Autodesk Inventor part; units mm, degrees
ref_plane "YZ Plane" through (0, 0, 0) normal (1, 0, 0) x (0, 1, 0)
ref_plane "XZ Plane" through (0, 0, 0) normal (0, 1, 0) x (-1, 0, 0)
ref_plane "XY Plane" through (0, 0, 0) normal (0, 0, 1) x (1, 0, 0)
sketch "Sketch1" plane through (0, 0, 0) normal (0, 0, 1) x (1, 0, 0)
  point P0 (0, 0)
sketch "0" plane through (0, 0, 0) normal (0, 0, 1) x (1, 0, 0)
  arc A0 (31.9, 54.31) -> (34.9, 51.31) centre (34.9, 54.31) ccw
  line L0 (34.9, 51.31) -> (39.9, 51.31)
  arc A1 (42.9, 48.31) -> (39.9, 51.31) centre (39.9, 48.31) ccw
  line L1 (42.9, 48.31) -> (42.9, 28.56)
  arc A2 (39.9, 25.56) -> (42.9, 28.56) centre (39.9, 28.56) ccw
  line L2 (39.9, 25.56) -> (34.9, 25.56)
  line L3 (15.6769, 19.4231) -> (14.5, 19.4231)
  arc A3 (12.5, 21.4231) -> (14.5, 19.4231) centre (14.5, 21.4231) ccw
  line L4 (12.5, 21.4231) -> (12.5, 22.56)
  arc A4 (12.5, 22.56) -> (9.5, 25.56) centre (9.5, 22.56) ccw
  line L5 (9.5, 51.31) -> (4.5, 51.31)
  arc A5 (4.5, 51.31) -> (1.5, 48.31) centre (4.5, 48.31) ccw
  line L6 (1.5, 48.31) -> (1.5, 28.56)
  arc A6 (1.5, 28.56) -> (4.5, 25.56) centre (4.5, 28.56) ccw
  line L7 (4.5, 25.56) -> (9.5, 25.56)
  arc A7 (31.9, 54.31) -> (28.9, 57.31) centre (28.9, 54.31) ccw
  line L8 (28.9, 57.31) -> (15.5, 57.31)
  arc A8 (15.5, 57.31) -> (12.5, 54.31) centre (15.5, 54.31) ccw
  line L9 (28.7231, 19.4231) -> (29.9, 19.4231)
  arc A9 (29.9, 19.4231) -> (31.9, 21.4231) centre (29.9, 21.4231) ccw
  line L10 (31.9, 21.4231) -> (31.9, 22.56)
  line L11 (12.705, 53.275) -> (12.705, 23.375)
  line L12 (15.805, 56.275) -> (28.595, 56.275)
  line L13 (31.595, 53.275) -> (31.595, 23.375)
  line L14 (30.345, 22.125) -> (14.055, 22.125)
  circle A10 centre (9.5, 54.31) radius 2
  circle A11 centre (9.5, 22.56) radius 2
  circle A12 centre (34.9, 22.56) radius 2
  circle A13 centre (34.9, 54.31) radius 2
  circle A14 centre (9.5, 54.31) radius 3
  circle A15 centre (9.5, 22.56) radius 3
  circle A16 centre (34.9, 22.56) radius 3
  circle A17 centre (34.9, 54.31) radius 3
  circle A18 centre (22.2, 12.9) radius 8.75
  circle A19 centre (22.2, 12.9) radius 9.225
  arc A20 (28.7231, 19.4231) -> (15.6769, 19.4231) centre (22.2, 12.9) ccw
  line L15 (22.2, 12.9) -> (28.7231, 19.4231)
  line L16 (22.2, 12.9) -> (31.425, 12.9)
  line L17 (22.2, 12.9) -> (15.6769, 19.4231)
  arc A21 (9.5, 51.31) -> (12.5, 54.31) centre (9.5, 54.31) ccw
  arc A22 (34.9, 25.56) -> (31.9, 22.56) centre (34.9, 22.56) ccw
  point P0 (31.9, 54.31)
  point P1 (12.5, 54.31)
  point P2 (4.5, 51.31)
  point P3 (1.5, 48.31)
extrude "Extrusion1" add sketch "0" along normal blind 1.5 contours A0 L0 A1 L1 A2 L2 A16 L10 A9 L9 A19 L3 A3 L4 A4 L7 A6 L6 A5 L5 A14 A8 L8 A7
properties part number "anchor-screen-cover"
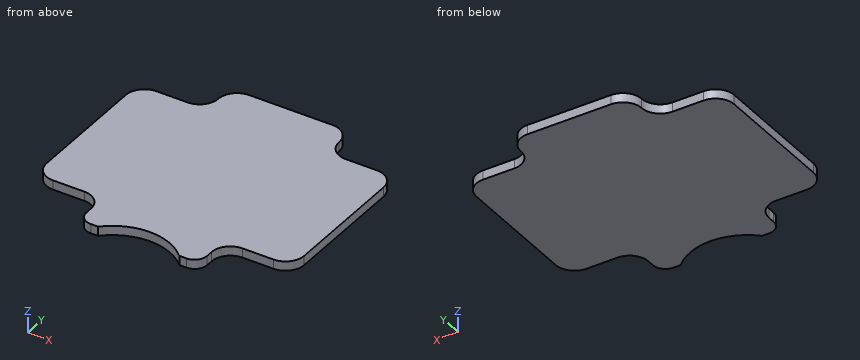
Can you work these out from the model? Positions are in its coordinate system, mm. Round coordinates to 2 decimals unless told otherwise and drop trailing zeros. Loops run counter-clockwise (first coordinate to the right, second up) from the corner with the lowest first, then second, coordinate; pieces in that order, holes last. Notation, with made-up numbers: (-21.75, -28) -> (36.25, -28) arc R25 ccw to (36.25, -3) -> close; hole circle Ø9 at (23, 51). An arc over 180 degrees is marked (long way). Answer in a Markdown table with one row per item.
Item 1: Suppose I cut it at C-C, the plane y = 50. List the corners of the cut face in (x, z) for me, plus the area to 3 significant figures.
Answer block:
| item | result |
|---|---|
| outline | (2.02, 0) -> (42.38, 0) -> (42.38, 1.5) -> (2.02, 1.5) -> close |
| area | 60.5 mm² |
Item 2: Suppose I cut it at B-B, the plane x = 8. List the corners of the cut face in (y, z) for me.
Answer block:
| item | result |
|---|---|
| outline | (25.56, 0) -> (51.31, 0) -> (51.31, 1.5) -> (25.56, 1.5) -> close |
Item 3: Will this pin go through, and if not, where does the flat tip stop? P1, Ø0.8, axis at x = 38, z = 0.5, coming from the +Y side.
Answer block:
| item | result |
|---|---|
| P1 | y = 51.31 |
Item 4: Suppose I cut it at A-A, the plane z = 1.2. List the corners of the cut face in (x, y) for me (3 decimals), plus the area to 3 significant figures.
Answer block:
| item | result |
|---|---|
| outline | (1.5, 28.56) arc R3 ccw to (4.5, 25.56) -> (9.5, 25.56) arc R3 cw to (12.5, 22.56) -> (12.5, 21.423) arc R2 ccw to (14.5, 19.423) -> (15.677, 19.423) arc R9.225 cw to (28.723, 19.423) -> (29.9, 19.423) arc R2 ccw to (31.9, 21.423) -> (31.9, 22.56) arc R3 cw to (34.9, 25.56) -> (39.9, 25.56) arc R3 ccw to (42.9, 28.56) -> (42.9, 48.31) arc R3 ccw to (39.9, 51.31) -> (34.9, 51.31) arc R3 cw to (31.9, 54.31) arc R3 ccw to (28.9, 57.31) -> (15.5, 57.31) arc R3 ccw to (12.5, 54.31) arc R3 cw to (9.5, 51.31) -> (4.5, 51.31) arc R3 ccw to (1.5, 48.31) -> close |
| area | 1,270 mm² |
Item 5: If I drill on probe 1 along Y at (x, z) = (36, 0.95); probe 2 along Y at (x, z) = (18, 0.5); probe 3 along X at (y, z) = (23, 0.8), over which ranges is the centre line in solid material (lowest first)?
Answer block:
| item | result |
|---|---|
| probe 1 | 25.56 to 51.31 |
| probe 2 | 21.11 to 57.31 |
| probe 3 | 12.47 to 31.93 |
